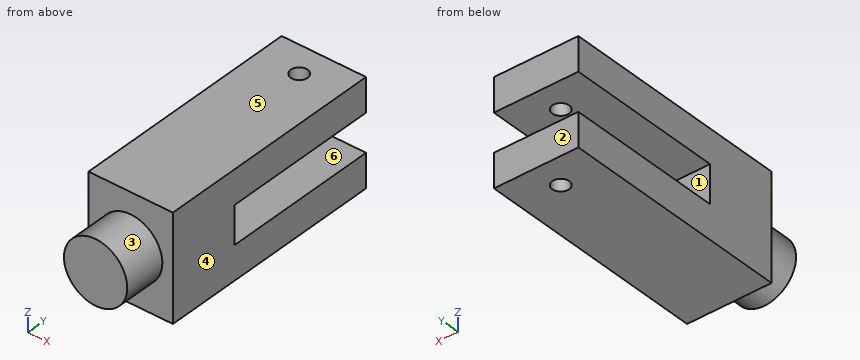
from build123d import *

# Parameters (mm, degrees)
SKETCH1_R           = 15
BOSS_EXTRUDE1_DEPTH = 20
SKETCH2_W           = 40
SKETCH2_H           = 50
BOSS_EXTRUDE2_DEPTH = 110
SKETCH3_W           = 18
SKETCH3_H           = 150
CUT_EXTRUDE1_DEPTH  = 139.293166859
SKETCH4_R           = 4
CUT_EXTRUDE2_DEPTH  = 141.712472795


with BuildPart() as part:
    # Sketch1 → Boss-Extrude1 (new body)
    with BuildSketch(Plane(origin=(0, 0, 0), x_dir=(1, 0, 0), z_dir=(0, 1, 0))):
        with Locations(Location((0, 0, 0), (0, 0, 270))):
            Circle(SKETCH1_R)
    extrude(amount=BOSS_EXTRUDE1_DEPTH)

    # Sketch2 → Boss-Extrude2 (add)
    with BuildSketch(Plane(origin=(0, 20, 0), x_dir=(1, 0, 0), z_dir=(0, 1, 0))):
        Rectangle(SKETCH2_W, SKETCH2_H)
    extrude(amount=BOSS_EXTRUDE2_DEPTH)

    # Sketch3 → Cut-Extrude1 (cut, through all)
    with BuildSketch(Plane(origin=(20, 0, 0), x_dir=(0, 0, -1), z_dir=(1, 0, 0))):
        with Locations((0, 130)):
            Rectangle(SKETCH3_W, SKETCH3_H)
    extrude(amount=-CUT_EXTRUDE1_DEPTH, mode=Mode.SUBTRACT)

    # Sketch4 → Cut-Extrude2 (cut, through all)
    with BuildSketch(Plane(origin=(0, 0, -25), x_dir=(-1, 0, 0), z_dir=(0, 0, -1))):
        with Locations((0, 116)):
            Circle(SKETCH4_R)
    extrude(amount=-CUT_EXTRUDE2_DEPTH, mode=Mode.SUBTRACT)


solid = part.part
The model under review builds one solid part; all positions refer to its coordinate system, in mm. Face numbers are marked on the shaded views. A direction names the side the tool comes from. Give positions to 0.01 mm unless a question says otherwise; leave off trailing zeros. Order: outer loops, then holes, each group sorted by start corner. A loop starts at its lowest first (then second) coordinate and runs counter-clockwise, first axis right, second up. Notation, with made-up numbers: M -34.5,75.5 L -27.5,75.5 A29 cw -27.5,105.5 Z; hole C 19.5,37 d1. An arc over 180 degrees is marked long. One line per question, with ' | ' between items. Start each with the question number.
1) Mouldability with a two-part tool opening along Z and no side actions: class the marked faces 4, 5 and 6 as pulls with the +Z half, pulls with the -Z half, needs draft (parallel to the pull), parting line crosses it, or undercut.
2) Wall thickness on L1, parallel to Z at x = 18, y = 93; L2, parallel to Y at x = 0, z = -13; L3, parallel to Y at x = 0, z = 17.75: over which ranges is each line inside the solid? List them lowest first. Write a range as from..to.
3) Clearance check with flat-ended pins moving along their axes: P1, Ø5.5, axis at x = -3, z = 0.5, coming from the +Y side; P2, Ø6.5, axis at x = 0, y = 116, coming from the +Z side. State where each tip first meets the part, or that it passes through.
4) For the marked faces 1, 2 and 3, list the 3-axis set-ups (+Z, -Z, +X, -X, +Y, -Y) from which the entire face can be reached by the end or side of a thin tool; tool diameter is ignored.
5) Consider section B-B, the plane y = 116. Give the boundary of the cut face in (x, z), then the cut area to 3 significant figures.
6) Consider section D-D, the plane x = -9. Give the boundary of the cut face in (y, z), then the cut area to 3 significant figures.
7) Consider section A-A, the plane x = 0. Give the boundary of the cut face in (y, z).
8) Consider section C-C, the plane z = 0. Give the boundary of the cut face in (x, y), then the cut area to 3 significant figures.
Found:
1) face 4: needs draft | face 5: pulls with the +Z half | face 6: undercut
2) L1: z = -25..-9, 9..25 | L2: y = 0..112, 120..130 | L3: y = 20..112, 120..130
3) P1: stops at y = 55 | P2: passes through
4) face 1: +X, -X, +Y | face 2: +Z, -Z, +X, -X, +Y | face 3: -Y
5) outline: M -20,-25 L -4,-25 L -4,-9 L -20,-9 Z; M -20,9 L -4,9 L -4,25 L -20,25 Z; M 4,-25 L 20,-25 L 20,-9 L 4,-9 Z; M 4,9 L 20,9 L 20,25 L 4,25 Z | area: 1,020 mm²
6) outline: M 0,-12 L 20,-12 L 20,-25 L 130,-25 L 130,-9 L 55,-9 L 55,9 L 130,9 L 130,25 L 20,25 L 20,12 L 0,12 Z | area: 4,630 mm²
7) outline: M 0,-15 L 20,-15 L 20,-25 L 112,-25 L 112,-9 L 55,-9 L 55,9 L 112,9 L 112,25 L 20,25 L 20,15 L 0,15 Z; M 120,-25 L 130,-25 L 130,-9 L 120,-9 Z; M 120,9 L 130,9 L 130,25 L 120,25 Z
8) outline: M -20,20 L -15,20 L -15,0 L 15,0 L 15,20 L 20,20 L 20,55 L -20,55 Z | area: 2,000 mm²
